Here's how the part is built. I have some questions about the finished solid (model axes, mm). Face numbers are marked on the shaded views. Give positions to 0.01 mm unless a question says otherwise; leave off trailing zeros. Loops run counter-clockwise (first coordinate to the right, second up) from the corner with the lowest first, then second, coordinate; pieces in that order, holes last. Notation, with made-up numbers: (72, 20.5) - (120, 20.5) arc R8 cw to (120, 30.5) - close; hole circle Ø9 at (-17.5, -9.5). An arc over 180 degrees is marked (long way). Use one line per item in the form item = value.
from build123d import *

# Parameters (mm, degrees)
F0_W      = 1778
F0_H      = 1016
F1_DEPTH  = 25.4
F2_W      = 76.2
F2_H      = 76.2
F3_DEPTH  = 717.55
F4_W      = 76.2
F4_H      = 368.3
F4_H_2    = 76.2
F5_DEPTH  = 19.05
F6_W      = 76.2
F6_H      = 368.3
F7_DEPTH  = 19.05
F9_DEPTH  = 76.2
F11_DEPTH = 76.2


with BuildPart() as f1:
    # F0 (on Top) → F1 (new body)
    with BuildSketch(Plane.XY):
        with Locations((891.739976, 508)):
            Rectangle(F0_W, F0_H)
    extrude(amount=F1_DEPTH)

    # F2 (on face) → F3 (join)
    with BuildSketch(Plane(origin=(0, 0, 0), x_dir=(1, 0, 0), z_dir=(0, 0, -1))):
        with Locations((269.439976, -508)):
            Rectangle(F2_W, F2_H)
        with Locations((1514.039976, -508)):
            Rectangle(F2_W, F2_H)
    extrude(amount=F3_DEPTH)

    # F4 (on face) → F5 (join)
    with BuildSketch(Plane(origin=(0, 0, -717.55), x_dir=(1, 0, 0), z_dir=(0, 0, -1))):
        with Locations((269.439976, -285.75)):
            Rectangle(F4_W, F4_H)
        with Locations((269.439976, -508)):
            Rectangle(F4_W, F4_H_2)
        with Locations((269.439976, -730.25)):
            Rectangle(F4_W, F4_H)
        with Locations((1514.039976, -285.75)):
            Rectangle(F4_W, F4_H)
        with Locations((1514.039976, -508)):
            Rectangle(F4_W, F4_H_2)
        with Locations((1514.039976, -730.25)):
            Rectangle(F4_W, F4_H)
    extrude(amount=F5_DEPTH)

    # F6 (on face) → F7 (join)
    with BuildSketch(Plane(origin=(0, 0, 0), x_dir=(1, 0, 0), z_dir=(0, 0, -1))):
        with Locations((1514.039976, -730.25)):
            Rectangle(F6_W, F6_H)
        with Locations((1514.039976, -285.75)):
            Rectangle(F6_W, F6_H)
        with Locations((269.439976, -730.25)):
            Rectangle(F6_W, F6_H)
        with Locations((269.439976, -285.75)):
            Rectangle(F6_W, F6_H)
    extrude(amount=F7_DEPTH)

    # F8 (on face) → F9 (join)
    with BuildSketch(Plane(origin=(231.339976, 0, 0), x_dir=(0, -1, 0), z_dir=(-1, 0, 0))):
        Polygon((-895.35, -19.05), (-546.1, -368.3), (-546.1, -260.536927), (-787.586927, -19.05), align=None)
        Polygon((-469.9, -368.3), (-120.65, -19.05), (-228.413073, -19.05), (-469.9, -260.536927), align=None)
        Polygon((-228.413073, -717.55), (-120.65, -717.55), (-469.9, -368.3), (-469.9, -476.063073), align=None)
        Polygon((-546.1, -476.063073), (-546.1, -368.3), (-895.35, -717.55), (-787.586927, -717.55), align=None)
    extrude(amount=-F9_DEPTH)

    # F10 (on face) → F11 (join)
    with BuildSketch(Plane.YZ.offset(1552.139976)):
        Polygon((120.65, -19.05), (469.9, -368.3), (469.9, -260.536927), (228.413073, -19.05), align=None)
        Polygon((546.1, -368.3), (895.35, -19.05), (787.586927, -19.05), (546.1, -260.536927), align=None)
        Polygon((787.586927, -717.55), (895.35, -717.55), (546.1, -368.3), (546.1, -476.063073), align=None)
        Polygon((469.9, -476.063073), (469.9, -368.3), (120.65, -717.55), (228.413073, -717.55), align=None)
    extrude(amount=-F11_DEPTH)


solid = f1.part
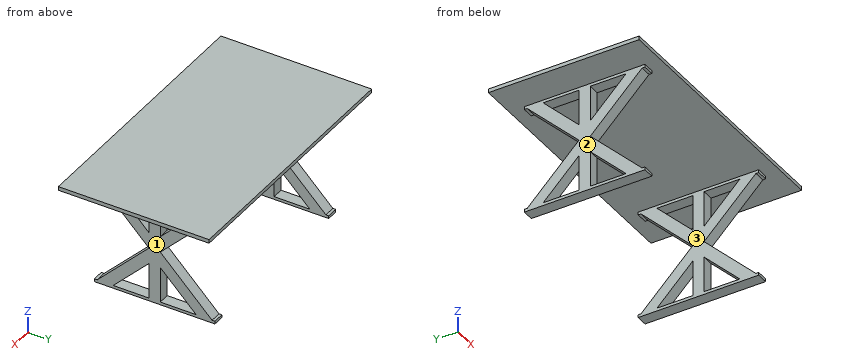
(1) If we section it at A-A (z = -312.5): List the corners of the cut face in (x, y) for me, plus the area to 3 significant figures.
Geometry says:
outline = (231.34, 414.1) - (307.54, 414.1) - (307.54, 601.9) - (231.34, 601.9) - close; (1475.94, 414.1) - (1552.14, 414.1) - (1552.14, 601.9) - (1475.94, 601.9) - close
area = 28,600 mm²
(2) If we section it at C-C (z = -213): List the corners of the cut face in (x, y) for me.
Geometry says:
outline = (231.34, 314.6) - (307.54, 314.6) - (307.54, 422.36) - (231.34, 422.36) - close; (231.34, 469.9) - (307.54, 469.9) - (307.54, 546.1) - (231.34, 546.1) - close; (231.34, 593.64) - (307.54, 593.64) - (307.54, 701.4) - (231.34, 701.4) - close; (1475.94, 314.6) - (1552.14, 314.6) - (1552.14, 422.36) - (1475.94, 422.36) - close; (1475.94, 469.9) - (1552.14, 469.9) - (1552.14, 546.1) - (1475.94, 546.1) - close; (1475.94, 593.64) - (1552.14, 593.64) - (1552.14, 701.4) - (1475.94, 701.4) - close
(3) If we section it at D-D (z = -442): List the corners of the cut face in (x, y) for me.
Geometry says:
outline = (231.34, 396.2) - (307.54, 396.2) - (307.54, 619.8) - (231.34, 619.8) - close; (1475.94, 396.2) - (1552.14, 396.2) - (1552.14, 619.8) - (1475.94, 619.8) - close
(4) For P1, Ø5, axis at y = 518, z = -608.5, coming from the +X side; P2, Ø21, axis at x = 1507, z = -731, coming from the +Y side; P3, Ø15, axis at x = 253.5, z = -726.5, coming from the -Y side, each with a flat end and sliding along its axis, tell me the tip position at first contact or that it passes through.
Geometry says:
P1 = 1552.14
P2 = 914.4
P3 = 101.6
(5) If we section it at B-B (y = 823.5): List the corners of the cut face in (x, z) for me, plus the area to 3 significant figures.
Geometry says:
outline = (2.74, 0) - (231.34, 0) - (231.34, -90.9) - (307.54, -90.9) - (307.54, 0) - (1475.94, 0) - (1475.94, -90.9) - (1552.14, -90.9) - (1552.14, 0) - (1780.74, 0) - (1780.74, 25.4) - (2.74, 25.4) - close; (231.34, -736.6) - (307.54, -736.6) - (307.54, -645.7) - (231.34, -645.7) - close; (1475.94, -736.6) - (1552.14, -736.6) - (1552.14, -645.7) - (1475.94, -645.7) - close
area = 72,900 mm²
(6) If I drill on probe 1 along Y at (x, z) = (1541.5, -233.5); probe 2 along X at (y, z) = (518.5, -87); probe 3 along Z at (x, y) = (151.5, 780.5), over which ranges is the centre line in solid material (lowest first)?
Geometry says:
probe_1 = 335.1 to 442.86, 469.9 to 546.1, 573.14 to 680.9
probe_2 = 231.34 to 307.54, 1475.94 to 1552.14
probe_3 = 0 to 25.4
(7) Thinking about a two-plate mould opening in X: for the marked faces 1, 2 and 3, which applies, pulls with the +X half, pulls with the -X half, needs draft (parallel to the pull), parting line crosses it, or undercut?
Geometry says:
face_1 = pulls with the +X half
face_2 = pulls with the -X half
face_3 = undercut
